Check sheet for the modelled part. Datum: model origin and axes. Units: mm. Face numbers are marked on the shaded views. A direction names the side the tool comes from. Round coordinates to 2 decimals unless told otherwise and drop trailing zeros. Write each loop counter-clockwise with the first axis right and the second up, starting at its lowest first coordinate (ties: lowest second). Pieces come first, ordered by that corner, then holes.
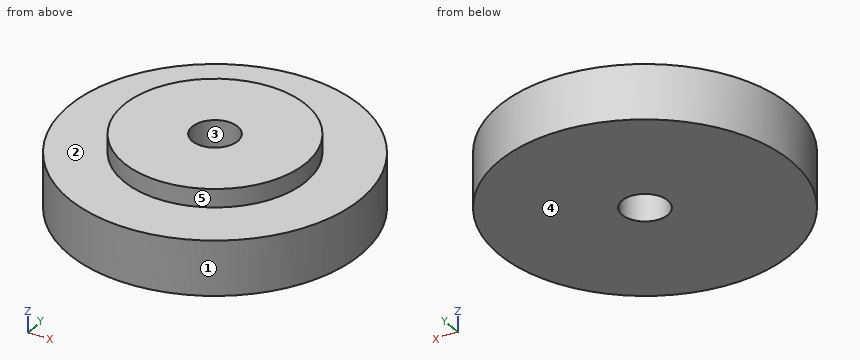
from build123d import *

# Parameters (mm, degrees)
F0_R     = 25.4
F1_DEPTH = 9.525
F2_R     = 15.875
F3_DEPTH = 3.175
F4_R     = 3.96875
F5_DEPTH = 12.701


with BuildPart() as f1:
    # F0 (on Top) → F1 (new body)
    with BuildSketch(Plane.XY):
        Circle(F0_R)
    extrude(amount=F1_DEPTH)

    # F2 (on face) → F3 (join)
    with BuildSketch(Plane.XY.offset(9.525)):
        Circle(F2_R)
    extrude(amount=F3_DEPTH)

    # F4 (on face) → F5 (cut, through all)
    with BuildSketch(Plane.XY.offset(12.7)):
        Circle(F4_R)
    extrude(amount=-F5_DEPTH, mode=Mode.SUBTRACT)


solid = f1.part
1. Scan lines: line 1 along Y through (x, z) = (0, 6.75); line 2 along Z through (x, y) = (19, -14.5) (3 decimals); line 3 along Y through (x, z) = (0, 10) (3 decimals). Record each from-to range of solid material in increasing order.
2. Set-up check for the marked faces 4 and 5: record each of +Z, -Z, +X, -X, +Y, -Y from which the full face is reachable in a straight line by a thin tool's end or side.
3. Sectioned sample at D-D, the plane y = 6. Enter the section's corners in (x, z) (3 decimals), plus the area to 3 significant figures.
4. Sectioned sample at A-A, the plane x = 0. Enter the section's corners in (y, z) (3 decimals), plus the area to 3 significant figures.
5. Release check for a two-part mould opening along X. For the marked faces 1, 2 and 3 record: released by +X, released by -X, zero draft, split by the parting line, or undercut.
6. Sectioned sample at C-C, the plane z = 8. Enter the section's corners in (x, y).
7. Go/stop test with flat-tipped pins: pin 1 (6 mm diameter, centred on x = -0.5, z = 2, fed in from -Y); pin 2 (1.5 mm diameter, centred on y = -11.5, z = 2.5, fed in from +X); pin 3 (1 mm diameter, centred on x = 12, z = 2.5, fed in from -Y). Record where each tip stops, or that it passes through.
Computed values:
1. line 1: y = -25.4 to -3.97, 3.97 to 25.4
1. line 2: z = 0 to 9.525
1. line 3: y = -15.875 to -3.969, 3.969 to 15.875
2. face 4: -Z, +X, -X, +Y, -Y
2. face 5: +Z
3. outline: (-24.681, 0) - (24.681, 0) - (24.681, 9.525) - (14.697, 9.525) - (14.697, 12.7) - (-14.697, 12.7) - (-14.697, 9.525) - (-24.681, 9.525) - close
3. area: 564 mm2
4. outline: (-25.4, 0) - (-3.969, 0) - (-3.969, 12.7) - (-15.875, 12.7) - (-15.875, 9.525) - (-25.4, 9.525) - close; (3.969, 0) - (25.4, 0) - (25.4, 9.525) - (15.875, 9.525) - (15.875, 12.7) - (3.969, 12.7) - close
4. area: 484 mm2
5. face 1: split by the parting line
5. face 2: zero draft
5. face 3: undercut
6. outline: circle Ø50.8 at (0, 0); hole circle Ø7.94 at (0, 0)
7. pin 1: stops at y = -25.4
7. pin 2: stops at x = 23.01
7. pin 3: stops at y = -22.65
